from build123d import *

# Parameters (mm, degrees)
SKETCH_1_R               = 3.1
SKETCH_1_R_2             = 2.1
EXTRUDE_1_DEPTH          = 3
CHAMFER_1_SIZE           = 2
CHAMFER_3_SIZE           = 4
CUT_EXTRUDE_1_DEPTH      = 146.124084838
CHAMFER_4_SIZE           = 3
CUT_EXTRUDE_2_DEPTH      = 146.124084838
PATTERN_CIRCULAR_1_COUNT = 3


with BuildPart() as part:
    # 草图1 → 凸台-拉伸1 (new, symmetric)
    with BuildSketch(Plane(origin=(0, 0, 0), x_dir=(1, 0, 0), z_dir=(0, 1, 0))):
        Polygon((-50, 100), (50, 100), (100, -45), (100, -105), (80, -105), (-100, -5), (-100, 55), align=None)
        with Locations(Location((0, 0, 0), (0, 0, 270))):
            Circle(SKETCH_1_R, mode=Mode.SUBTRACT)
        with Locations(Location((-20, 90, 0), (0, 0, 270))):
            Circle(SKETCH_1_R_2, mode=Mode.SUBTRACT)
        with Locations(Location((-90, 45, 0), (0, 0, 270))):
            Circle(SKETCH_1_R_2, mode=Mode.SUBTRACT)
        with Locations(Location((-90, 5, 0), (0, 0, 270))):
            Circle(SKETCH_1_R_2, mode=Mode.SUBTRACT)
        with Locations(Location((20, 90, 0), (0, 0, 90))):
            Circle(SKETCH_1_R_2, mode=Mode.SUBTRACT)
        with Locations(Location((90, -55, 0), (0, 0, 270))):
            Circle(SKETCH_1_R_2, mode=Mode.SUBTRACT)
        with Locations(Location((90, -95, 0), (0, 0, 270))):
            Circle(SKETCH_1_R_2, mode=Mode.SUBTRACT)
    extrude(amount=EXTRUDE_1_DEPTH, both=True)

    # 倒角1
    chamfer_1_edges = [part.edges().sort_by_distance(p)[0] for p in [
        (-20, -3, -92.1),
        (-90, -3, -47.1),
        (-90, -3, -7.1),
        (90, -3, 52.9),
        (90, -3, 92.9),
        (20, -3, -87.9),
    ]]
    chamfer(chamfer_1_edges, length=CHAMFER_1_SIZE)

    # 倒角3
    chamfer_3_edges = [part.edges().sort_by_distance(p)[0] for p in [
        (100, 0, 105),
    ]]
    chamfer(chamfer_3_edges, length=CHAMFER_3_SIZE)

    # 草图2 → 切除-拉伸1 (cut, through all)
    with BuildSketch(Plane(origin=(0, 3, 0), x_dir=(1, 0, 0), z_dir=(0, 1, 0))):
        with BuildLine():
            Line((-78.344823658, 54.309222637), (-51.225659109, 78.716470731))
            ThreePointArc((-51.225659109, 78.716470731), (-44.16436472, 78.344823658), (-44.536011793, 71.283529269))
            Line((-44.536011793, 71.283529269), (-71.655176342, 46.876281175))
            ThreePointArc((-71.655176342, 46.876281175), (-78.716470731, 47.247928248), (-78.344823658, 54.309222637))
        make_face()
        with BuildLine():
            Line((70.669187988, -36.629953417), (32.738153505, 73.370046583))
            ThreePointArc((32.738153505, 73.370046583), (35.835064997, 79.726864908), (42.191883322, 76.629953417))
            Line((42.191883322, 76.629953417), (80.122917804, -33.370046583))
            ThreePointArc((80.122917804, -33.370046583), (77.026006313, -39.726864908), (70.669187988, -36.629953417))
        make_face()
        with BuildLine():
            Line((67.571785344, -80.936052734), (-72.428214656, -3.158274956))
            ThreePointArc((-72.428214656, -3.158274956), (-74.370786381, 3.64072608), (-67.571785344, 5.583297805))
            Line((-67.571785344, 5.583297805), (72.428214656, -72.194479973))
            ThreePointArc((72.428214656, -72.194479973), (74.370786381, -78.993481009), (67.571785344, -80.936052734))
        make_face()
    extrude(amount=-CUT_EXTRUDE_1_DEPTH, mode=Mode.SUBTRACT)

    # 倒角4
    chamfer_4_edges = [part.edges().sort_by_distance(p)[0] for p in [
        (0, -3, -3.1),
    ]]
    chamfer(chamfer_4_edges, length=CHAMFER_4_SIZE)

    # 草图3 → 切除-拉伸2 (cut, through all)
    with BuildSketch(Plane.XZ.offset(3)):
        with BuildLine():
            ThreePointArc((12.277060504, -26.328241213), (16.662395476, -23.796366887), (20.541451993, -20.541451993))
            ThreePointArc((20.541451993, -20.541451993), (20.541451993, -14.813887066), (14.813887066, -14.813887066))
            ThreePointArc((14.813887066, -14.813887066), (12.016426342, -17.161235328), (8.853852583, -18.987148138))
            ThreePointArc((8.853852583, -18.987148138), (6.894910006, -24.369298636), (12.277060504, -26.328241213))
        make_face()
    cut_extrude_2 = extrude(amount=-CUT_EXTRUDE_2_DEPTH, mode=Mode.SUBTRACT)

    # 阵列(圆周)1: 切除-拉伸2 ×3 about axis
    pattern_circular_1_axis = Axis((0, 0, 0), (0, 1, 0))
    for i in range(1, PATTERN_CIRCULAR_1_COUNT):
        add(cut_extrude_2.rotate(pattern_circular_1_axis, i * 360 / PATTERN_CIRCULAR_1_COUNT), mode=Mode.SUBTRACT)


solid = part.part
The listing builds one solid part. Answer for the finished solid, in the listing's coordinates (mm). A direction names the side the tool comes from. Coordinates: 2 decimals unless noted, no trailing zeros. Loops run counter-clockwise (first coordinate to the right, second up) from the corner with the lowest first, then second, coordinate; pieces in that order, holes last. Notation, with made-up numbers: (40, 21.5) -> (94, 21.5) arc R21 ccw to (94, 58.5) -> close; hole circle Ø3 at (-12, 85). An arc over 180 degrees is marked (long way). Write item = value, one per line. Start each with the question number.
1) Given pin 1 Ø1 at (x, y) = (-36.5, -1) entering from +Z; pin 2 Ø2 at (y, z) = (-0.5, -32) entering from +X; pin 3 Ø5 at (x, z) = (-90, -45) entering from -Y, each flat-ended and moving along its own axis, determine where each tip first touches the part or whether it passes through.
2) A cutting plane is placed at A-A (x = 0). Give the vertices of the cut face in (y, z).
3) Straight lines are drawn through the part: line 1 (X direction, y = 0.75, z = -0.5); line 2 (X direction, y = -2, z = -62); line 3 (Z direction, x = -17.5, y = -1.75). For each, find the intervals that lie inside material, in ascending order. Write a range as from..to.
4) The mould has two halves that part along X. Classify faces 1 (the face through (1, -3, -22)), 2 (the face through (-8.74, 0.04, 55.7)), 3 (the face through (-19.902, -1.125, -92.223)), 4 (the face through (-92.172, -1.125, -5.482)): released by +X, released by -X, zero draft, split by the parting line, or undercut.
5) A cutting plane is placed at B-B (x = 59). Give the vertices of the cut face in (y, z).
6) A tool of negligible diameter and unlimited length cuts with its end or side. For faces 5 (the face through (-100, 0, -25)), 6 (the face through (16.6, -0.04, -23.84)), from which of +Z, -Z, +X, -X, +Y, -Y can it reach the whole face along a straight path? Write none if from no direction.
Responses:
q1.pin_1 = 40.56
q1.pin_2 = 73.79
q1.pin_3 = -1.4
q2.outline = (-3, -100) -> (3, -100) -> (3, -3.1) -> (0, -3.1) -> (-3, -6.1) -> close; (-3, 6.1) -> (0, 3.1) -> (3, 3.1) -> (3, 31.96) -> (-3, 31.96) -> close; (-3, 43.4) -> (3, 43.4) -> (3, 60.56) -> (-3, 60.56) -> close
q3.line_1 = -100..-74.95, -58.42..-29.05, -20.94..-3.06, 3.06..57.87, 68.44..84.31
q3.line_2 = -92.22..-69.8, -54.85..36.66, 47.24..63.1
q3.line_3 = -100..-91.37, -88.63..22.23, 33.67..50.83
q4.face_1 = zero draft
q4.face_2 = released by -X
q4.face_3 = undercut
q4.face_4 = undercut
q5.outline = (-3, -73.9) -> (3, -73.9) -> (3, -27.89) -> (-3, -27.89) -> close; (-3, 2.79) -> (3, 2.79) -> (3, 64.73) -> (-3, 64.73) -> close; (-3, 76.17) -> (3, 76.17) -> (3, 93.33) -> (-3, 93.33) -> close
q6.face_5 = +Z, -Z, -X, +Y, -Y
q6.face_6 = +Y, -Y
